from build123d import *

# Parameters (mm, degrees)
SKETCH3_W           = 965.2
SKETCH3_H           = 508
BOSS_EXTRUDE2_DEPTH = 101.6
SKETCH4_R           = 25.4
CUT_EXTRUDE2_DEPTH  = 101.6
SKETCH7_W           = 152.4
SKETCH7_H           = 50.8
BOSS_EXTRUDE4_DEPTH = 152.4
SKETCH10_R          = 19.05
CUT_EXTRUDE3_DEPTH  = 609.6


with BuildPart() as part:
    # Sketch3 → Boss-Extrude2 (new body)
    with BuildSketch(Plane(origin=(0, 0, 0), x_dir=(0, 0, -1), z_dir=(1, 0, 0))):
        with Locations((232.546367736, 490.753272684)):
            Rectangle(SKETCH3_W, SKETCH3_H)
    extrude(amount=BOSS_EXTRUDE2_DEPTH)

    # Sketch4 → Cut-Extrude2 (cut)
    with BuildSketch(Plane(origin=(0, 0, 0), x_dir=(0, 0, -1), z_dir=(1, 0, 0))):
        with Locations((-151.217224275, 681.253272684)):
            Circle(SKETCH4_R)
        with Locations((-162.181898332, 300.253272684)):
            Circle(SKETCH4_R)
    extrude(amount=CUT_EXTRUDE2_DEPTH, mode=Mode.SUBTRACT)

    # Sketch7 → Boss-Extrude4 (add)
    with BuildSketch(Plane(origin=(0, 0, 0), x_dir=(0, 0, -1), z_dir=(1, 0, 0))):
        with Locations((638.946367736, 490.753272684)):
            Rectangle(SKETCH7_W, SKETCH7_H)
    extrude(amount=BOSS_EXTRUDE4_DEPTH)

    # Sketch10 → Cut-Extrude3 (cut)
    with BuildSketch(Plane(origin=(0, 0, 0), x_dir=(1, 0, 0), z_dir=(0, 1, 0))):
        with Locations(Location((127, 638.946367736, 0), (0, 0, 90))):
            Circle(SKETCH10_R)
    extrude(amount=CUT_EXTRUDE3_DEPTH, mode=Mode.SUBTRACT)


solid = part.part
Part model, mm, in its own coordinate system. A direction names the side the tool comes from. Round coordinates to 2 decimals unless told otherwise and drop trailing zeros. Write each loop counter-clockwise with the first axis right and the second up, starting at its lowest first coordinate (ties: lowest second). Pieces come first, ordered by that corner, then holes. Notation, with made-up numbers: M 11.5,-30.5 L 45.5,-30.5 A31 ccw 45.5,7.5 Z; hole C -23,27 d2. An arc over 180 degrees is marked long. Return JSON: item names as keys, results as strings. Group by question number.
(1) Two-plate mould, pull along Z, no slides. Class faces 5 (the face through (50.1, 277.7, 150.5)), 6 (the face through (0, 494, -226)), 7 (the face through (58, 487, -715.146)): +Z half, -Z half, draft (parallel to the pull), parting line (faces both ways), or undercut.
(2) Drill centre lines: probe 1 along X at (y, z) = (324, -510.5); probe 2 along Y at (x, z) = (76.5, 166); probe 3 along Z at (x, y) = (65.5, 694.5). Where is each one in solid material? Low to high.
(3) Which spindle directions (+Z, -Z, +X, -X, +Y, -Y) get a long thin tool onto all of the face, cutting with end or side? Do faces 1 (the face through (152.4, 491, -638)), 2 (the face through (138, 465.353, -621)), 3 (the face through (127, 490, -562.746)), 4 (the face through (138, 516.153, -621)). Say none if no direction does.
(4) Saw through at C-C on z = -269. Write the cut outline in (x, y).
(5) Pin check, flat tips, straight feed: pin 1 Ø1.5 at (y, z) = (617.5, 18) entering from +X; pin 2 Ø15 at (x, z) = (115, -607.5) entering from -Y. Stop position of each tip, or through.
(6) Saw through at B-B on y = 598.5. Write the cut outline in (x, z).
(7) Saw through at A-A on x = 127. Write the cut outline in (y, z), then the cut area to 3 significant figures.
Returned:
{
 "1": {"face 5": "undercut", "face 6": "draft", "face 7": "-Z half"},
 "2": {"probe 1": "0 to 101.6", "probe 2": "236.75 to 275.14, 325.36 to 660.6, 701.91 to 744.75", "probe 3": "-715.15 to 129.55, 172.89 to 250.05"},
 "3": {"face 1": "+Z, -Z, +X, +Y, -Y", "face 2": "+Z, -Z, +X, -Y", "face 3": "+Z, +X, +Y, -Y", "face 4": "+Z, -Z, +X, +Y"},
 "4": {"outline": "M 0,236.75 L 101.6,236.75 L 101.6,744.75 L 0,744.75 Z"},
 "5": {"pin 1": "x = 101.6", "pin 2": "y = 465.35"},
 "6": {"outline": "M 0,-715.15 L 101.6,-715.15 L 101.6,250.05 L 0,250.05 Z"},
 "7": {"outline": "M 465.35,-715.15 L 516.15,-715.15 L 516.15,-658 L 465.35,-658 Z; M 465.35,-619.9 L 516.15,-619.9 L 516.15,-562.75 L 465.35,-562.75 Z", "area": "5,810 mm²"}
}
